Can you work these out from the model? Positions are in its coordinate system, mm. Give positions to 0.01 mm unless a question says otherwise; leave off trailing zeros. Write each loop counter-clockwise with the first axis right and the second up, starting at its lowest first coordinate (ties: lowest second). Pieces come first, ordered by that corner, then holes.
```python
from build123d import *

# Parameters (mm, degrees)
SKETCH_1_W         = 252.1
SKETCH_1_H         = 84
EXTRUDE_1_DEPTH    = 1
SKETCH1_R          = 1.5
CUT_EXTRUDE1_DEPTH = 10
SKETCH4_R          = 7.4
CUT_EXTRUDE3_DEPTH = 133.878149069
SKETCH5_R          = 1.5
CUT_EXTRUDE4_DEPTH = 10


with BuildPart() as part:
    # 草图1 → 凸台-拉伸1 (new, symmetric)
    with BuildSketch(Plane(origin=(0, 0, 0), x_dir=(1, 0, 0), z_dir=(0, 1, 0))):
        Rectangle(SKETCH_1_W, SKETCH_1_H)
    extrude(amount=EXTRUDE_1_DEPTH, both=True)

    # Sketch1 → Cut-Extrude1 (cut)
    with BuildSketch(Plane(origin=(0, 1, 0), x_dir=(1, 0, 0), z_dir=(0, 1, 0))):
        with Locations(Location((-122.05, 36.25, 0), (0, 0, 270))):
            Circle(SKETCH1_R)
        with Locations(Location((-122.05, -36.25, 0), (0, 0, 270))):
            Circle(SKETCH1_R)
        with Locations(Location((122.05, -36.25, 0), (0, 0, 270))):
            Circle(SKETCH1_R)
        with Locations(Location((122.05, 36.25, 0), (0, 0, 270))):
            Circle(SKETCH1_R)
    extrude(amount=-CUT_EXTRUDE1_DEPTH, mode=Mode.SUBTRACT)

    # Sketch4 → Cut-Extrude3 (cut, through all)
    with BuildSketch(Plane(origin=(0, 1, 0), x_dir=(1, 0, 0), z_dir=(0, 1, 0))):
        with Locations(Location((-111.05, 19, 0), (0, 0, 270))):
            Circle(SKETCH4_R)
        with Locations(Location((111.05, 19, 0), (0, 0, 270))):
            Circle(SKETCH4_R)
    extrude(amount=-CUT_EXTRUDE3_DEPTH, mode=Mode.SUBTRACT)

    # Sketch5 → Cut-Extrude4 (cut)
    with BuildSketch(Plane(origin=(0, 1, 0), x_dir=(1, 0, 0), z_dir=(0, 1, 0))):
        with Locations(Location((-111.05, 1.5, 0), (0, 0, 270))):
            Circle(SKETCH5_R)
        with Locations(Location((-111.05, 36.5, 0), (0, 0, 270))):
            Circle(SKETCH5_R)
        with Locations(Location((111.05, 1.5, 0), (0, 0, 270))):
            Circle(SKETCH5_R)
        with Locations(Location((111.05, 36.5, 0), (0, 0, 270))):
            Circle(SKETCH5_R)
    extrude(amount=-CUT_EXTRUDE4_DEPTH, mode=Mode.SUBTRACT)


solid = part.part
```
1) Suppose I cut it at A-A on y = -0.4. State how many separate pieces and enclosed holes the cut face has, plus the area to 3 significant figures.
Values follow:
separate pieces: 1
enclosed holes: 10
area: 20,800 mm2
2) Suppose I cut it at B-B on z = -21. Write out the boundary of the cut face in (x, y), plus the area to 3 significant figures.
Values follow:
outline: (-126.05, -1) - (-118.17, -1) - (-118.17, 1) - (-126.05, 1) - close; (-103.93, -1) - (103.93, -1) - (103.93, 1) - (-103.93, 1) - close; (118.17, -1) - (126.05, -1) - (126.05, 1) - (118.17, 1) - close
area: 447 mm2
3) Please list where these lines run through material, in increasing order: L1, parallel to X at y = -0.05, z = -1.5; L2, parallel to X at y = -0.4, z = 36.25; L3, parallel to X at y = 0, z = -36.25.
Values follow:
L1: x = -126.05 to -112.55, -109.55 to 109.55, 112.55 to 126.05
L2: x = -126.05 to -123.55, -120.55 to 120.55, 123.55 to 126.05
L3: x = -126.05 to -123.55, -120.55 to -112.53, -109.57 to 109.57, 112.53 to 120.55, 123.55 to 126.05
4) For pin 1 Ø2.5 at (x, z) = (122.05, -36.25) entering from +Y, with a flat end and sliding along its axis, tell me the tip position at first contact or that it passes through.
Values follow:
pin 1: passes through
5) If we mould it in two halves opening along Z, with no side actions, what happens to faces 1 (the face through (-2, -1, -1)), 2 (the face through (103.826, 0.014, -20.604)), 3 (the face through (-118.274, 0.014, -20.604))? For each: +Z half, -Z half, draft (parallel to the pull), parting line (faces both ways), or undercut.
Values follow:
face 1: draft
face 2: undercut
face 3: undercut
